```python
from build123d import *

# Parameters (mm, degrees)
SKETCH2_W           = 14
SKETCH2_H           = 14.003492138
BOSS_EXTRUDE1_DEPTH = 2


with BuildPart() as part:
    # Sketch2 → Boss-Extrude1 (new body)
    with BuildSketch(Plane(origin=(0, 0, 0), x_dir=(1, 0, 0), z_dir=(0, 1, 0))):
        with BuildLine():
            Line((-1095.769577908, -1082.63934327), (-1107.541983277, -1061.584764794))
            ThreePointArc((-1107.541983277, -1061.584764794), (-1108.000297721, -1058.999800443), (-1106.757289889, -1056.687437072))
            Line((-1106.757289889, -1056.687437072), (-1095.359092699, -1050.106684856))
            ThreePointArc((-1095.359092699, -1050.106684856), (-1093.52896568, -1048.276557838), (-1092.859092699, -1045.776557838))
            Line((-1092.859092699, -1045.776557838), (-1094.115480669, -1009.711041726))
            ThreePointArc((-1094.115480669, -1009.711041726), (-1093.777019534, -1007.720622139), (-1092.679112618, -1006.026241285))
            ThreePointArc((-1092.679112618, -1006.026241285), (-1032.311467942, -988.369881675), (-985.507730543, -1030.38666075))
            ThreePointArc((-985.507730543, -1030.38666075), (-985.278073332, -1031.364982485), (-985.24860148, -1032.369466065))
            Line((-985.24860148, -1032.369466065), (-985.404903488, -1034.555701493))
            Line((-985.404903488, -1034.555701493), (-990.945620353, -1073.979950898))
            ThreePointArc((-990.945620353, -1073.979950898), (-992.753308552, -1076.67957505), (-995.991887306, -1076.939026078))
            ThreePointArc((-995.991887306, -1076.939026078), (-1043.957441778, -1071.676478665), (-1090.53391343, -1084.286835898))
            ThreePointArc((-1090.53391343, -1084.286835898), (-1093.478902478, -1084.502780598), (-1095.769577908, -1082.63934327))
        make_face()
        Polygon((-1086.294602377, -1012.058273794), (-1072.303130777, -1011.569680794), (-1071.814676576, -1025.557177729), (-1085.806148176, -1026.045770729), align=None, mode=Mode.SUBTRACT)
        Polygon((-1068.720871477, -999.537331894), (-1068.232278477, -1013.528803494), (-1054.244579364, -1013.040342232), (-1054.733172364, -999.048870632), align=None, mode=Mode.SUBTRACT)
        Polygon((-1050.906333977, -993.912186894), (-1036.914862377, -993.423593894), (-1036.426243752, -1007.415799297), (-1050.417715352, -1007.904392297), align=None, mode=Mode.SUBTRACT)
        Polygon((-1027.613440377, -999.372618594), (-1013.632626977, -1000.105321994), (-1014.36558899, -1014.091070024), (-1028.34640239, -1013.358366624), align=None, mode=Mode.SUBTRACT)
        Polygon((-1028.503151677, -1016.349320694), (-1014.522338277, -1017.082024094), (-1015.25503736, -1031.062755126), (-1029.23585076, -1030.330051726), align=None, mode=Mode.SUBTRACT)
        Polygon((-1029.392862977, -1033.326022794), (-1015.412049577, -1034.058726194), (-1016.144804819, -1048.04052879), (-1030.125618219, -1047.30782539), align=None, mode=Mode.SUBTRACT)
        Polygon((-1007.457654877, -1032.332416694), (-993.593901877, -1034.280840094), (-995.542405578, -1048.145164464), (-1009.406158578, -1046.196741064), align=None, mode=Mode.SUBTRACT)
        Polygon((-1050.313042577, -1010.901830994), (-1036.321570977, -1010.413237994), (-1035.832862611, -1024.408013247), (-1049.824334211, -1024.896606247), align=None, mode=Mode.SUBTRACT)
        Polygon((-1068.127580077, -1016.526975994), (-1054.136108477, -1016.038382994), (-1053.647579498, -1030.028021263), (-1067.639051098, -1030.516614263), align=None, mode=Mode.SUBTRACT)
        Polygon((-1067.534288677, -1033.516620094), (-1053.542817077, -1033.028027094), (-1053.054129332, -1047.022211839), (-1067.045600932, -1047.510804839), align=None, mode=Mode.SUBTRACT)
        Polygon((-1085.701310977, -1029.047917894), (-1071.709839377, -1028.559324894), (-1071.22126078, -1042.550384043), (-1085.21273238, -1043.038977043), align=None, mode=Mode.SUBTRACT)
        Polygon((-1049.719751177, -1027.891475094), (-1035.728279577, -1027.402882094), (-1035.239810651, -1041.390800691), (-1049.231282251, -1041.879393691), align=None, mode=Mode.SUBTRACT)
        with Locations((-1046.973178577, -1058.907162363)):
            Rectangle(SKETCH2_W, SKETCH2_H, mode=Mode.SUBTRACT)
        Polygon((-1076.546392677, -1056.655668794), (-1063.023431077, -1053.032202194), (-1059.399339813, -1066.557495071), (-1072.922301413, -1070.180961671), align=None, mode=Mode.SUBTRACT)
        Polygon((-1099.786325567, -1062.934815358), (-1092.78632559, -1075.059170971), (-1080.661053874, -1068.058642082), (-1087.661053851, -1055.934286468), align=None, mode=Mode.SUBTRACT)
    extrude(amount=BOSS_EXTRUDE1_DEPTH)


solid = part.part
```
CAD build for the part. Positions are in the model's coordinates, mm. A direction names the side the tool comes from. Round coordinates to 2 decimals unless told otherwise and drop trailing zeros. Write each loop counter-clockwise with the first axis right and the second up, starting at its lowest first coordinate (ties: lowest second). Pieces come first, ordered by that corner, then holes. Notation, with made-up numbers: (-31, 68.5) -> (6, 68.5) arc R29 cw to (6, 94.5) -> close; hole circle Ø6 at (-27, 1.25). An arc over 180 degrees is marked (long way). Answer in a Markdown table with one row per item. Add a question column.
Item 1: Drop flat-ended pins along their axis: pin 1 Ø3 at (x, z) = (-1043, 1008) entering from -Y; pin 2 Ø1 at (x, y) = (-1045, 1.5) entering from +Z; pin 3 Ø0.6 at (y, z) = (1, 1055.5) entering from -X. Give the stop position or say it passes through.
Item 2: Saw through at A-A, the plane z = 996. Write the cut outline in (x, y).
Item 3: Saw through at B-B, the plane x = -1046. Write the cut outline in (y, z), then the cut area to 3 significant figures.
Item 4: Saw through at C-C, the plane z = 1023. Write the cut outline in (x, y), then the cut area to 3 significant figures.
Item 5: Drill centre lines: line 1 (X direction, y = 1, z = 1010); line 2 (X direction, y = 1.8, z = 1011); line 3 (Z direction, x = -1045, y = 0.55). Where is each one in solid material? Low to high. Write a range as from..to.
Item 6: Mould opens along X. For faces 4 (the face through (-1046, 2, 1046)), 5 (the face through (-988.136, 0.986, 1053.992)), 6 (the face through (-1084.1, 1, 1062.1)) say: pulls with the +X half, pulls with the -X half, needs draft (parallel to the pull), parting line crosses it, or undercut.
Item 7: Which spindle directions (+Z, -Z, +X, -X, +Y, -Y) get a long thin tool onto all of the face, cutting with end or side? Do faces 1 (the face through (-1093.55, 0.99, 1048.31)), 2 (the face through (-1093.639, 0.986, 1059.386)), 3 (the face through (-1043.28, 0.986, 1071.626)). Say none if no direction does.
Item 8: Saw through at D-D, the plane y = 1.05. Count the separate pieces of the cut face and the enclosed holes in it, then the cut area to 3 significant figures.
Findings below:
| question | item | result |
|---|---|---|
| 1 | pin 1 | stops at y = 0 |
| 1 | pin 2 | stops at z = 1071.81 |
| 1 | pin 3 | stops at x = -1105.22 |
| 2 | outline | (-1079.94, 0) -> (-1050.83, 0) -> (-1050.83, 2) -> (-1079.94, 2) -> close; (-1036.82, 0) -> (-1013.34, 0) -> (-1013.34, 2) -> (-1036.82, 2) -> close |
| 3 | outline | (0, 986.77) -> (2, 986.77) -> (2, 993.74) -> (0, 993.74) -> close; (0, 1007.75) -> (2, 1007.75) -> (2, 1010.75) -> (0, 1010.75) -> close; (0, 1024.76) -> (2, 1024.76) -> (2, 1027.76) -> (0, 1027.76) -> close; (0, 1041.77) -> (2, 1041.77) -> (2, 1051.91) -> (0, 1051.91) -> close; (0, 1065.91) -> (2, 1065.91) -> (2, 1071.85) -> (0, 1071.85) -> close |
| 3 | area | 58.1 mm^2 |
| 4 | outline | (-1093.65, 0) -> (-1085.91, 0) -> (-1085.91, 2) -> (-1093.65, 2) -> close; (-1071.9, 0) -> (-1067.9, 0) -> (-1067.9, 2) -> (-1071.9, 2) -> close; (-1053.89, 0) -> (-1049.89, 0) -> (-1049.89, 2) -> (-1053.89, 2) -> close; (-1035.88, 0) -> (-1028.85, 0) -> (-1028.85, 2) -> (-1035.88, 2) -> close; (-1014.83, 0) -> (-988.57, 0) -> (-988.57, 2) -> (-1014.83, 2) -> close |
| 4 | area | 98.1 mm^2 |
| 5 | line 1 | x = -1094.11..-1068.36, -1054.35..-1028.17, -1014.15..-997 |
| 5 | line 2 | x = -1094.07..-1068.32, -1054.32..-1050.31, -1036.3..-1028.22, -1014.2..-996.18 |
| 5 | line 3 | z = 986.78..993.71, 1007.72..1010.72, 1024.73..1027.73, 1041.73..1051.91, 1065.91..1071.76 |
| 6 | face 4 | needs draft |
| 6 | face 5 | pulls with the +X half |
| 6 | face 6 | undercut |
| 7 | face 1 | -X, +Y, -Y |
| 7 | face 2 | +Y, -Y |
| 7 | face 3 | +Z, +Y, -Y |
| 8 | separate pieces | 1 |
| 8 | enclosed holes | 15 |
| 8 | area | 5,760 mm^2 |
